```python
from build123d import *

# Parameters (mm, degrees)
ESBO_O2_W                = 140
ESBO_O2_H                = 200
RESSALTO_EXTRUS_O2_DEPTH = 4
ESBO_O11_W               = 2
ESBO_O11_H               = 4
RESSALTO_EXTRUS_O3_DEPTH = 69
RESSALTO_EXTRUS_O4_DEPTH = 69
ESBO_O14_W               = 140
ESBO_O14_H               = 4
RESSALTO_EXTRUS_O5_DEPTH = 175
ESBO_O17_W               = 140
ESBO_O17_H               = 6
RESSALTO_EXTRUS_O6_DEPTH = 10
ESBO_O18_W               = 140
ESBO_O18_H               = 6
CORTE_EXTRUS_O1_DEPTH    = 10


with BuildPart() as part:
    # Esboço2 → Ressalto-extrusão2 (new body)
    with BuildSketch(Plane.XY):
        Rectangle(ESBO_O2_W, ESBO_O2_H)
    extrude(amount=RESSALTO_EXTRUS_O2_DEPTH)

    # Varredura1: sweep along a curve in space
    with BuildLine() as varredura1_path:
        Line((0, -98, 0), (0, -47.285808591, -108.756934444))
    # Esboço11 → Varredura1 (sweep)
    with BuildSketch(Plane.XY.offset(-108.756934444)):
        with Locations((0, -47.285808591)):
            Rectangle(ESBO_O11_W, ESBO_O11_H)
    sweep(path=varredura1_path.line)

    # Esboço12 → Ressalto-extrusão3 (add)
    with BuildSketch(Plane(origin=(1, 0, 0), x_dir=(0, 0, -1), z_dir=(1, 0, 0))):
        Polygon((108.756934444, -45.285808591), (0, -96), (0, -100), (108.756934444, -49.285808591), align=None)
    extrude(amount=RESSALTO_EXTRUS_O3_DEPTH)

    # Esboço13 → Ressalto-extrusão4 (add)
    with BuildSketch(Plane.ZY.offset(1)):
        Polygon((-108.756934444, -49.285808591), (0, -100), (0, -96), (-108.756934444, -45.285808591), align=None)
    extrude(amount=RESSALTO_EXTRUS_O4_DEPTH)

    # Esboço14 → Ressalto-extrusão5 (add)
    with BuildSketch(Plane(origin=(0, -78.853805265, -36.77013327), x_dir=(1, 0, 0), z_dir=(0, 0.906307787036648, 0.4226182617407039))):
        with Locations((0, 37.428646873)):
            Rectangle(ESBO_O14_W, ESBO_O14_H)
    extrude(amount=RESSALTO_EXTRUS_O5_DEPTH)

    # Esboço17 → Ressalto-extrusão6 (add)
    with BuildSketch(Plane.XY.offset(4)):
        with Locations((0, 93.234832477)):
            Rectangle(ESBO_O17_W, ESBO_O17_H)
    extrude(amount=RESSALTO_EXTRUS_O6_DEPTH)

    # Esboço18 → Corte-extrusão1 (cut)
    with BuildSketch(Plane.XY.offset(14)):
        with Locations((0, 93.234832477)):
            Rectangle(ESBO_O18_W, ESBO_O18_H)
    extrude(amount=-CORTE_EXTRUS_O1_DEPTH, mode=Mode.SUBTRACT)


solid = part.part
```
Source: CAD feature listing. Evaluate the final solid. Frame: model axes, mm. A direction names the side the tool comes from. Give positions to 0.01 mm unless a question says otherwise; leave off trailing zeros. Write each loop counter-clockwise with the first axis right and the second up, starting at its lowest first coordinate (ties: lowest second). Pieces come first, ordered by that corner, then holes.
1. Material intervals for line 1 along Z through (x, y) = (-19.5, -57); line 2 along Z through (x, y) = (28, 34); line 3 along Z through (x, y) = (-28, -24), sorted ascending.
2. Section query C-C (z = -55). Return the cut outline in (x, y).
3. Section query A-A (y = -70). Return the cut outline in (x, z).
4. Section query B-B (x = -49). Return the cut outline in (y, z).
5. Pull-direction query (Z, two-part tool) for faces 6 (the face through (0.98, -80.165, -33.958)), 7 (the face through (0.98, -74.29, -55.14)), 8 (the face through (-70, 0, -40)); classes: +Z half, -Z half, draft (parallel to the pull), parting line (faces both ways), or undercut.
6. First-contact query: pin 1 (4 mm diameter, centred on x = -52, z = -53.5, fed in from +Y); pin 2 (2 mm diameter, centred on x = -30, z = -11.5, fed in from +Y); pin 3 (1.5 mm diameter, centred on x = -2.5, z = -75.5, fed in from -Y). Flat tips, straight axial feed; report the tip coordinate or a pass-through.
7. Access query for faces 1 (the face through (-1, 1, 4)), 2 (the face through (70, 0, -40)), 3 (the face through (-1, -5, 0)), 4 (the face through (-1, 97, 0)), 5 (the face through (0.98, -53.857, -90.377)). Directions: +Z, -Z, +X, -X, +Y, -Y. A direction counts if a zero-diameter tool reaches every point of the face in a straight line with its end or side. Return the directions, or none.
8. Section query D-D (z = -81). Return the cut outline in (x, y), then the cut area to 3 significant figures.
Output values:
1. line 1: z = -92.21 to -83.64, -70.08 to -65.67, 0 to 4
1. line 2: z = -27.65 to -23.24, 0 to 4
1. line 3: z = -54.7 to -50.28, 0 to 4
2. outline: (-70, -74.35) - (70, -74.35) - (70, -70.35) - (-70, -70.35) - close; (-70, -34.12) - (70, -34.12) - (70, -24.65) - (-70, -24.65) - close
3. outline: (-70, -64.34) - (70, -64.34) - (70, -55.76) - (-70, -55.76) - close; (-70, 0) - (70, 0) - (70, 4) - (-70, 4) - close
4. outline: (-100, 0) - (-49.29, -108.76) - (-45.29, -108.76) - (-62.19, -72.5) - (93.3, 0) - (100, 0) - (100, 4) - (-100, 4) - close; hole (-96, 0) - (-63.88, -68.88) - (83.83, 0) - close
5. face 6: undercut
5. face 7: -Z half
5. face 8: draft
6. pin 1: stops at y = -17.15
6. pin 2: stops at y = 70.78
6. pin 3: stops at y = -65.14
7. face 1: +Z, +X, -X, +Y, -Y
7. face 2: +Z, -Z, +X, +Y, -Y
7. face 3: +X, -X
7. face 4: -Z, +X, -X, +Y
7. face 5: +X, -X, +Y
8. outline: (-70, -62.23) - (70, -62.23) - (70, -58.23) - (-70, -58.23) - close
8. area: 560 mm2
